Input: part model. Units: mm. Frame: model coordinates. A direction names the side the tool comes from. Give positions to 0.01 mm unless a question says otherwise; leave off trailing zeros. Order: outer loops, then holes, each group sorted by start corner. A loop starts at its lowest first (then second) coordinate and runs counter-clockwise, first axis right, second up.
```python
from build123d import *

# Parameters (mm, degrees)
SKETCH1_R           = 11
BOSS_EXTRUDE1_DEPTH = 10
SKETCH2_R           = 2.1
CUT_EXTRUDE1_DEPTH  = 10
FILLET2_R           = 18
FILLET3_R           = 30
FILLET4_R           = 34
FILLET7_R           = 3


with BuildPart() as part:
    # Sketch1 → Boss-Extrude1 (new body)
    with BuildSketch(Plane(origin=(0, 0, 0), x_dir=(1, 0, 0), z_dir=(0, 1, 0))):
        with BuildLine():
            Line((-43.837879331, 11.61), (-37.199459056, 10.61))
            Line((-37.199459056, 10.61), (-3.38, 25.61))
            Line((-3.38, 25.61), (7.395945787, 26.61))
            Line((7.395945787, 26.61), (12.62, 28.528895207))
            ThreePointArc((12.62, 28.528895207), (29.66875295, -0.102896427), (13.12, -29.026558802))
            Line((13.12, -29.026558802), (7.395945787, -26.89))
            Line((7.395945787, -26.89), (-3.38, -25.89))
            Line((-3.38, -25.89), (-41.837879331, -11.39))
            Line((-41.837879331, -11.39), (-43.837879331, 11.61))
        make_face()
        with Locations(Location((-3.38, -0.39, 0), (0, 0, 270))):
            Circle(SKETCH1_R, mode=Mode.SUBTRACT)
    extrude(amount=BOSS_EXTRUDE1_DEPTH)

    # Sketch2 → Cut-Extrude1 (cut)
    with BuildSketch(Plane(origin=(0, 10, 0), x_dir=(1, 0, 0), z_dir=(0, 1, 0))):
        with Locations(Location((12.42, 2.131904043, 0), (0, 0, 270))):
            Circle(SKETCH2_R)
        with Locations(Location((-0.858095957, -16.19, 0), (0, 0, 270))):
            Circle(SKETCH2_R)
        with Locations(Location((-19.18, -2.911904043, 0), (0, 0, 270))):
            Circle(SKETCH2_R)
        with Locations(Location((-5.901904043, 15.41, 0), (0, 0, 270))):
            Circle(SKETCH2_R)
    extrude(amount=-CUT_EXTRUDE1_DEPTH, mode=Mode.SUBTRACT)

    # Fillet1
    # an asymmetric fillet: 18, 12 mm, written as the material it takes off along each edge
    with BuildSketch(Plane(origin=(-41.837879331, -35.518473591, 11.39), x_dir=(0.9357013977145019, 0, 0.3527929907397927), z_dir=(0, 1, 0))) as fillet1_piece_1:
        with BuildLine():
            Bezier((4.674389222, 0), (0, 0), (-6.145067451, 12.809686203), weights=[1, 0.846323269, 1])
            Line((-6.145067451, 12.809686203), (0, 0))
            Line((0, 0), (4.674389222, 0))
        make_face()
    extrude(amount=81.036947182, mode=Mode.SUBTRACT)

    # Fillet2
    fillet2_edges = [part.edges().sort_by_distance(p)[0] for p in [
        (-37.199459056, 5, -10.61),
    ]]
    fillet(fillet2_edges, radius=FILLET2_R)

    # Fillet3
    fillet3_edges = [part.edges().sort_by_distance(p)[0] for p in [
        (-3.38, 5, -25.61),
        (-3.38, 5, 25.89),
    ]]
    fillet(fillet3_edges, radius=FILLET3_R)

    # Fillet4
    fillet4_edges = [part.edges().sort_by_distance(p)[0] for p in [
        (7.395945787, 5, -26.61),
        (7.395945787, 5, 26.89),
    ]]
    fillet(fillet4_edges, radius=FILLET4_R)

    # Fillet7
    fillet7_edges = [part.edges().sort_by_distance(p)[0] for p in [
        (12.62, 5, -28.528895207),
        (13.12, 5, 29.026558802),
    ]]
    fillet(fillet7_edges, radius=FILLET7_R)


solid = part.part
```
1) Cut plane D-D (z = -21). Return the cut outline in (x, y), then the cut area to 3 significant figures.
2) Cut plane C-C (y = 8.75). Count the separate pieces of the cut face and the enclosed holes in it, then the cut area to 3 significant figures.
3) Line query: probe 1 along Z at (x, y) = (-4.5, 7); probe 2 along X at (y, z) = (7.75, 3.5); probe 3 along Z at (x, y) = (-5.5, 5.25). Output: solid intervals per line, ascending.
4) First-contact query: P1, Ø1.5, axis at y = 4, z = 6.5, coming from the +X side; P2, Ø1.5, axis at x = -11.5, y = 7.5, coming from the +Z side. Flat tips, straight axial feed; report the tip coordinate or a pass-through.
5) Reachability of faces 4 (the face through (-43.1, 4.9, -11.5)), 5 (the face through (-22.1, 4.93, 18.83)) from +Z, -Z, +X, -X, +Y, -Y: full face, straight path, thin tool, end or side. Return the list, or none.
6) Pull-direction query (Z, two-part tool) for faces 1 (the face through (13.14, 5.07, 28.69)), 2 (the face through (-1.66, 5.07, 18.13)), 3 (the face through (29.66, 4.93, -0.39)); classes: pulls with the +Z half, pulls with the -Z half, needs draft (parallel to the pull), parting line crosses it, or undercut.
7) Cut plane B-B (x = -19.18). Return the cut outline in (y, z), then the cut area to 3 significant figures.
8) Cut plane A-A (z = 15.5). Return the cut outline in (x, y).
Geometry says:
1. outline: (-13.77, 0) - (21.81, 0) - (21.81, 10) - (-13.77, 10) - close
1. area: 356 mm2
2. separate pieces: 1
2. enclosed holes: 5
2. area: 2,510 mm2
3. probe 1: z = -24.88 to -16.97, -13.85 to -10.55, 11.33 to 25.33
3. probe 2: x = -42.19 to -21.2, -17.16 to -13.93, 7.17 to 29.52
3. probe 3: z = -24.55 to -17.47, -13.35 to -10.4, 11.18 to 25.04
4. P1: stops at x = 29.23
4. P2: stops at z = 23.11
5. face 4: -Z, +Y, -Y
5. face 5: +Z, -X, +Y, -Y
6. face 1: pulls with the +Z half
6. face 2: undercut
6. face 3: parting line crosses it
7. outline: (0, -18.6) - (10, -18.6) - (10, 0.81) - (0, 0.81) - close; (0, 5.01) - (10, 5.01) - (10, 19.93) - (0, 19.93) - close
7. area: 343 mm2
8. outline: (-30.94, 0) - (-2.84, 0) - (-2.84, 10) - (-30.94, 10) - close; (1.13, 0) - (26.01, 0) - (26.01, 10) - (1.13, 10) - close
